```python
from build123d import *

# Parameters (mm, degrees)
F0_W         = 914.4
F0_H         = 304.8
F1_DEPTH     = 304.8
F2_T         = -6.35
F3_R         = 5.08
F4_T1_DEPTH  = 307.34
F4_T3_DEPTH  = 904.24
F4_T5_DEPTH  = 294.64
F4_S9_W      = 5.1816
F4_S9_H      = 5.1816
F4_T10_DEPTH = 5.1816
F4_S15_W     = 5.1816
F4_S15_H     = 5.1816
F4_T16_DEPTH = 5.1816
F4_S21_W     = 5.1816
F4_S21_H     = 5.1816
F4_T22_DEPTH = 5.1816
F4_S27_W     = 5.1816
F4_S27_H     = 5.1816
F4_T28_DEPTH = 5.1816


# Not quite as in the source:
# - a fillet or chamfer that OpenCascade refuses, or shapes differently, is made with other operations: its cross-section is extruded or revolved along the edge and cut away or added


with BuildPart() as f1:
    # F0 (on Front) → F1 (new body)
    with BuildSketch(Plane.XZ):
        with Locations((-4.9767009914, -156.8363738472)):
            Rectangle(F0_W, F0_H)
    extrude(amount=F1_DEPTH)

    # F2
    f2_openings = [f1.faces().sort_by_distance(p)[0] for p in [
        (-4.976701, -304.8, -156.836374),
    ]]
    offset(amount=F2_T, openings=f2_openings)

    # F3
    f3_edges = [f1.edges().sort_by_distance(p)[0] for p in [
        (-4.976701, -304.8, -4.436374),
        (-462.176701, -304.8, -156.836374),
        (-4.976701, -304.8, -309.236374),
        (452.223299, -304.8, -156.836374),
    ]]
    fillet(f3_edges, radius=F3_R)

    # F4: fillet of radius 5.08 on 12 edges, made by hand

    # F4_s2 → F4_t1 (cut)
    with BuildSketch(Plane.XZ.offset(5.08)):
        with BuildLine():
            ThreePointArc((452.2232990086, -9.5163738472), (450.735401457, -5.9242713988), (447.1432990086, -4.4363738472))
            Line((447.1432990086, -4.4363738472), (452.2232990086, -4.4363738472))
            Line((452.2232990086, -4.4363738472), (452.2232990086, -9.5163738472))
        make_face()
        with BuildLine():
            ThreePointArc((-457.0967009914, -4.4363738472), (-460.6888034398, -5.9242713988), (-462.1767009914, -9.5163738472))
            Line((-462.1767009914, -9.5163738472), (-462.1767009914, -4.4363738472))
            Line((-462.1767009914, -4.4363738472), (-457.0967009914, -4.4363738472))
        make_face()
        with BuildLine():
            ThreePointArc((-457.0967009914, -309.2363738472), (-460.6888034398, -307.7484762956), (-462.1767009914, -304.1563738472))
            Line((-462.1767009914, -304.1563738472), (-462.1767009914, -309.2363738472))
            Line((-462.1767009914, -309.2363738472), (-457.0967009914, -309.2363738472))
        make_face()
        with BuildLine():
            ThreePointArc((452.2232990086, -304.1563738472), (450.735401457, -307.7484762956), (447.1432990086, -309.2363738472))
            Line((447.1432990086, -309.2363738472), (452.2232990086, -309.2363738472))
            Line((452.2232990086, -309.2363738472), (452.2232990086, -304.1563738472))
        make_face()
    extrude(amount=F4_T1_DEPTH, mode=Mode.SUBTRACT)

    # F4_s4 → F4_t3 (cut)
    with BuildSketch(Plane.YZ.offset(-457.0967009914)):
        with BuildLine():
            ThreePointArc((0, -9.5163738472), (-1.4878975516, -5.9242713988), (-5.08, -4.4363738472))
            Line((-5.08, -4.4363738472), (0, -4.4363738472))
            Line((0, -4.4363738472), (0, -9.5163738472))
        make_face()
        with BuildLine():
            ThreePointArc((-5.08, -309.2363738472), (-1.4878975516, -307.7484762956), (0, -304.1563738472))
            Line((0, -304.1563738472), (0, -309.2363738472))
            Line((0, -309.2363738472), (-5.08, -309.2363738472))
        make_face()
    extrude(amount=F4_T3_DEPTH, mode=Mode.SUBTRACT)

    # F4_s6 → F4_t5 (cut)
    with BuildSketch(Plane.XY.offset(-304.1563738472)):
        with BuildLine():
            ThreePointArc((-457.0967009914, 0), (-460.6888034398, -1.4878975516), (-462.1767009914, -5.08))
            Line((-462.1767009914, -5.08), (-462.1767009914, 0))
            Line((-462.1767009914, 0), (-457.0967009914, 0))
        make_face()
        with BuildLine():
            ThreePointArc((452.2232990086, -5.08), (450.735401457, -1.4878975516), (447.1432990086, 0))
            Line((447.1432990086, 0), (452.2232990086, 0))
            Line((452.2232990086, 0), (452.2232990086, -5.08))
        make_face()
    extrude(amount=F4_T5_DEPTH, mode=Mode.SUBTRACT)


with BuildPart() as f4_tool8:
    # F4_s9 → F4_t10 (new body)
    with BuildSketch(Plane.YZ.offset(447.1432990086)):
        with Locations((-2.4892, -6.9255738472)):
            Rectangle(F4_S9_W, F4_S9_H)
    extrude(amount=F4_T10_DEPTH)

    # F4_s11 → F4_t12 (revolve, cut)
    with BuildSketch(Plane(origin=(447.1432990086, -5.08, -9.5163738472), x_dir=(0, -0.7071067812, -0.7071067812), z_dir=(0, -0.7071067812, 0.7071067812))):
        with BuildLine():
            ThreePointArc((0, -5.08), (5.08, 0), (0, 5.08))
            Line((0, 5.08), (0, -5.08))
        make_face()
    revolve(axis=Axis((447.1432990086, -5.08, -9.5163738472), (1, 0, 0)), mode=Mode.SUBTRACT)


with BuildPart() as f1_1:
    add(f1.part)

    # F4_t7: cut F4_tool8
    add(f4_tool8.part, mode=Mode.SUBTRACT)


with BuildPart() as f4_tool14:
    # F4_s15 → F4_t16 (new body)
    with BuildSketch(Plane.XZ.offset(5.08)):
        with Locations((-459.6875009914, -6.9255738472)):
            Rectangle(F4_S15_W, F4_S15_H)
    extrude(amount=-F4_T16_DEPTH)

    # F4_s17 → F4_t18 (revolve, cut)
    with BuildSketch(Plane(origin=(-457.0967009914, -5.08, -9.5163738472), x_dir=(0.7071067812, 0, -0.7071067812), z_dir=(0.7071067812, 0, 0.7071067812))):
        with BuildLine():
            ThreePointArc((0, -5.08), (5.08, 0), (0, 5.08))
            Line((0, 5.08), (0, -5.08))
        make_face()
    revolve(axis=Axis((-457.0967009914, -5.08, -9.5163738472), (0, 1, 0)), mode=Mode.SUBTRACT)


with BuildPart() as f1_2:
    add(f1_1.part)

    # F4_t13: cut F4_tool14
    add(f4_tool14.part, mode=Mode.SUBTRACT)


with BuildPart() as f4_tool20:
    # F4_s21 → F4_t22 (new body)
    with BuildSketch(Plane.XY.offset(-304.1563738472)):
        with Locations((-459.6875009914, -2.4892)):
            Rectangle(F4_S21_W, F4_S21_H)
    extrude(amount=-F4_T22_DEPTH)

    # F4_s23 → F4_t24 (revolve, cut)
    with BuildSketch(Plane(origin=(-457.0967009914, -5.08, -304.1563738472), x_dir=(0.7071067812, -0.7071067812, 0), z_dir=(0.7071067812, 0.7071067812, 0))):
        with BuildLine():
            ThreePointArc((0, -5.08), (5.08, 0), (0, 5.08))
            Line((0, 5.08), (0, -5.08))
        make_face()
    revolve(axis=Axis((-457.0967009914, -5.08, -304.1563738472), (0, 0, -1)), mode=Mode.SUBTRACT)


with BuildPart() as f1_3:
    add(f1_2.part)

    # F4_t19: cut F4_tool20
    add(f4_tool20.part, mode=Mode.SUBTRACT)


with BuildPart() as f4_tool26:
    # F4_s27 → F4_t28 (new body)
    with BuildSketch(Plane.YZ.offset(447.1432990086)):
        with Locations((-2.4892, -306.7471738472)):
            Rectangle(F4_S27_W, F4_S27_H)
    extrude(amount=F4_T28_DEPTH)

    # F4_s29 → F4_t30 (revolve, cut)
    with BuildSketch(Plane(origin=(447.1432990086, -5.08, -304.1563738472), x_dir=(0, -0.7071067812, 0.7071067812), z_dir=(0, 0.7071067812, 0.7071067812))):
        with BuildLine():
            ThreePointArc((0, -5.08), (5.08, 0), (0, 5.08))
            Line((0, 5.08), (0, -5.08))
        make_face()
    revolve(axis=Axis((447.1432990086, -5.08, -304.1563738472), (1, 0, 0)), mode=Mode.SUBTRACT)


with BuildPart() as f1_4:
    add(f1_3.part)

    # F4_t25: cut F4_tool26
    add(f4_tool26.part, mode=Mode.SUBTRACT)


solid = f1_4.part
```
Could you check a few things on this model? Use its own coordinates, in mm. A direction names the side the tool comes from. Coordinates: 2 decimals unless noted, no trailing zeros. Write each loop counter-clockwise with the first axis right and the second up, starting at its lowest first coordinate (ties: lowest second). Pieces come first, ordered by that corner, then holes. Notation, with made-up numbers: (-6, -28) -> (32, -28) arc R19 cw to (32, -4) -> close; hole circle Ø2 at (54.25, 20). An arc over 180 degrees is marked (long way). One line per question, with ' | ' between items. Start each with the question number.
1. For faces 1 (the face through (-11, -150, -4.436)), 2 (the face through (-11, -153, -10.786)), which set-ups out of +Z, -Z, +X, -X, +Y, -Y let a thin tool reach every point of the face, with its end or its side?
2. If we section it at A-A (x = 295): Please give me the cut outline in (y, z), and give its area (3 significant figures).
3. Thinking about a two-plate mould opening in Z: for faces 3 (the face through (-11, -150, -309.236)), 4 (the face through (-11, 0, -155)), 5 (the face through (-11, -6.35, -155)), 6 (the face through (-455.827, -153, -159)), which applies, pulls with the +Z half, pulls with the -Z half, needs draft (parallel to the pull), parting line crosses it, or undercut?
4. Please list where these lines run through material, in increasing order: line 1 along X through (y, z) = (-159, -246.5); line 2 along Z through (x, y) = (153.5, -25); line 3 along Y through (x, z) = (267, -174).
5. Will this pin go through, and if not, where does the flat tip stop? P1, Ø1.5, axis at x = -306.5, z = -259.5, coming from the -Y side.
6. If we section it at C-C (z = -235): Please give me the cut outline in (x, y), and give its area (3 significant figures).
7. If we section it at B-B (y = -166): Please give me the cut outline in (x, z), and give its area (3 significant figures).
Return value:
1) face 1: +Z, +X, -X, +Y, -Y | face 2: -Y
2) outline: (-304.8, -304.16) arc R5.08 ccw to (-299.72, -309.24) -> (-5.08, -309.24) arc R5.08 ccw to (0, -304.16) -> (0, -9.52) arc R5.08 ccw to (-5.08, -4.44) -> (-299.72, -4.44) arc R5.08 ccw to (-304.8, -9.52) -> (-304.8, -10.79) -> (-6.35, -10.79) -> (-6.35, -302.89) -> (-304.8, -302.89) -> close | area: 5,700 mm²
3) face 3: pulls with the -Z half | face 4: needs draft | face 5: undercut | face 6: undercut
4) line 1: x = -462.18 to -455.83, 445.87 to 452.22 | line 2: z = -309.24 to -302.89, -10.79 to -4.44 | line 3: y = -6.35 to 0
5) P1: stops at y = -6.35
6) outline: (-462.18, -299.72) arc R5.08 ccw to (-457.1, -304.8) -> (-455.83, -304.8) -> (-455.83, -6.35) -> (445.87, -6.35) -> (445.87, -304.8) -> (447.14, -304.8) arc R5.08 ccw to (452.22, -299.72) -> (452.22, -5.08) arc R5.08 ccw to (447.14, 0) -> (-457.1, 0) arc R5.08 ccw to (-462.18, -5.08) -> close | area: 9,570 mm²
7) outline: (-462.18, -304.16) arc R5.08 ccw to (-457.1, -309.24) -> (447.14, -309.24) arc R5.08 ccw to (452.22, -304.16) -> (452.22, -9.52) arc R5.08 ccw to (447.14, -4.44) -> (-457.1, -4.44) arc R5.08 ccw to (-462.18, -9.52) -> close; hole (-455.83, -302.89) -> (445.87, -302.89) -> (445.87, -10.79) -> (-455.83, -10.79) -> close | area: 15,300 mm²
